```python
from build123d import *

# Parameters (mm, degrees)
BOSS_EXTRUDE1_DEPTH     = 400
CUT_EXTRUDE2_DEPTH      = 1
CUT_EXTRUDE2_DEPTH_BACK = 1311.69690242
SKETCH4_W               = 95
SKETCH4_H               = 10
CUT_EXTRUDE3_DEPTH      = 109


with BuildPart() as part:
    # Sketch1 → Boss-Extrude1 (new body)
    with BuildSketch(Plane(origin=(0, 0, 0), x_dir=(0, 0, -1), z_dir=(1, 0, 0))):
        Polygon((0, 0), (-340, 0), (-350, 10), (-350, 960), (-310, 1000), (-203.251091608, 1000), (-203.251091608, 1310.69690242), (-108.48888922, 1310.69690242), (0, 1310.69690242), (0, 1000), (0, 970), (0, 820), (-9.396926208, 806.579798567), (-27.474774195, 800), (-190.603073792, 740.62615458), (-200, 727.205953147), (-200, 5), (0, 5), align=None)
    extrude(amount=BOSS_EXTRUDE1_DEPTH)

    # Sketch3 → Cut-Extrude2 (cut, two sides)
    with BuildSketch(Plane(origin=(0, 0, 0), x_dir=(-1, 0, 0), z_dir=(0, -1, 0))) as cut_extrude2_sk:
        Polygon((32.971910004, -72.804395349), (-67.728153305, 29.569560354), (-322.648629759, 29.569560354), (-423.348693067, -72.804395349), (-423.348693067, 100.069531779), (32.971910004, 100.069531779), align=None)
    extrude(amount=CUT_EXTRUDE2_DEPTH, mode=Mode.SUBTRACT)
    extrude(cut_extrude2_sk.sketch, amount=-CUT_EXTRUDE2_DEPTH_BACK, mode=Mode.SUBTRACT)

    # Sketch4 → Cut-Extrude3 (cut)
    with BuildSketch(Plane.XY.offset(350)):
        with Locations((200, 895)):
            Rectangle(SKETCH4_W, SKETCH4_H)
    extrude(amount=-CUT_EXTRUDE3_DEPTH, mode=Mode.SUBTRACT)


solid = part.part
```
Could you check a few things on this model? Use its own coordinates, in mm. A direction names the side the tool comes from. Coordinates: 2 decimals unless noted, no trailing zeros. Write each loop counter-clockwise with the first axis right and the second up, starting at its lowest first coordinate (ties: lowest second). Pieces come first, ordered by that corner, then holes. Notation, with made-up numbers: (-19, 4) -> (-12, 4) arc R22 cw to (-12, 32) -> close; hole circle Ø1 at (-14.5, 53). An arc over 180 degrees is marked (long way). Return JSON: item names as keys, results as strings.
(1) Imagine slicing it at D-D, the plane x = 205. Please give me the cut outline in (y, z), then the cut area to 3 significant figures.
Numbers:
{"outline": "(0, 0) -> (5, 0) -> (5, 200) -> (727.21, 200) -> (740.63, 190.6) -> (806.58, 9.4) -> (820, 0) -> (1310.7, 0) -> (1310.7, 203.25) -> (1000, 203.25) -> (1000, 310) -> (960, 350) -> (900, 350) -> (900, 241) -> (890, 241) -> (890, 350) -> (10, 350) -> (0, 340) -> close", "area": "257,000 mm2"}
(2) Imagine slicing it at B-B, the plane y = 206.5. Please give me the cut outline in (x, z), then the cut area to 3 significant figures.
Numbers:
{"outline": "(0, 200) -> (400, 200) -> (400, 350) -> (0, 350) -> close", "area": "60,000 mm2"}
(3) Which directions (+Z, -Z, +X, -X, +Y, -Y) give clear straight access to the entire face, cutting with the end or side of a thin tool? Please do faces 4 (the flat face through (197, 1000, 257)), 5 (the flat face through (197, 371, 200)), 6 (the flat face through (197, 1310.697, 100)), 7 (the flat face through (199, 890, 296)).
Numbers:
{"face 4": "+Z, +X, -X, +Y", "face 5": "-Z, +X, -X", "face 6": "+Z, -Z, +X, -X, +Y", "face 7": "+Z"}
(4) I'm going to push flat-ended pins straight in: pin 1 (3 mm diameter, centred on x = 160, y = 234, fed in from -Z); pin 2 (5 mm diameter, centred on x = 139, z = 223, fed in from +Y). Where does each tip first touch, or does it pass through?
Numbers:
{"pin 1": "stops at z = 200", "pin 2": "stops at y = 1000"}
(5) We'd pull the mould along Y, two halves only. Please class faces 1 (the flat face through (197, 980, 330)), 2 (the flat face through (199, 900, 296)), 3 (the flat face through (197, 1153, 203.251)): +Y half, -Y half, draft (parallel to the pull), parting line (faces both ways), or undercut.
Numbers:
{"face 1": "+Y half", "face 2": "undercut", "face 3": "draft"}
(6) Imagine slicing it at A-A, the plane x = 97. Please give me the cut outline in (y, z), then the cut area to 3 significant figures.
Numbers:
{"outline": "(0, 0) -> (5, 0) -> (5, 200) -> (727.21, 200) -> (740.63, 190.6) -> (806.58, 9.4) -> (820, 0) -> (1310.7, 0) -> (1310.7, 203.25) -> (1000, 203.25) -> (1000, 310) -> (960, 350) -> (10, 350) -> (0, 340) -> close", "area": "259,000 mm2"}
(7) Imagine slicing it at C-C, the plane z = 216. Please give me the cut outline in (x, y), then the cut area to 3 significant figures.
Numbers:
{"outline": "(0, 0) -> (400, 0) -> (400, 1000) -> (0, 1000) -> close", "area": "400,000 mm2"}
(8) I need wall thicknesses on L1, parallel to X at y = 893, z = 314; L2, parallel to Z at x = 252, y = 233.5; L3, parallel to Y at x = 119, z = 307.5. Which ranges of each line are inside material? Lowest first, please.
Numbers:
{"L1": "x = 0 to 152.5, 247.5 to 400", "L2": "z = 200 to 350", "L3": "y = 0 to 1000"}
